from build123d import *

# Parameters (mm, degrees)
BOSS_EXTRUDE1_DEPTH = 10
CUT_EXTRUDE1_DEPTH  = 56.837607918
SKETCH3_R           = 2
CUT_EXTRUDE2_DEPTH  = 3
CUT_EXTRUDE3_DEPTH  = 1.5
FILLET1_R           = 3


with BuildPart() as part:
    # Sketch1 → Boss-Extrude1 (new body)
    with BuildSketch(Plane(origin=(0, 0, 0), x_dir=(0, 0, -1), z_dir=(1, 0, 0))):
        Polygon((0, 0), (0, 45), (31.509339219, 0), align=None)
    extrude(amount=-BOSS_EXTRUDE1_DEPTH)

    # Sketch2 → Cut-Extrude1 (cut, through all)
    with BuildSketch(Plane(origin=(0, 0, 0), x_dir=(0, 0, -1), z_dir=(1, 0, 0))):
        Polygon((25.746392839, 3), (3, 35.485215593), (3, 3), align=None)
    extrude(amount=-CUT_EXTRUDE1_DEPTH, mode=Mode.SUBTRACT)

    # Sketch3 → Cut-Extrude2 (cut)
    with BuildSketch(Plane.XZ):
        with Locations(Location((-5, -8, 0), (0, 0, 270))):
            Circle(SKETCH3_R)
        with Locations(Location((-5, -16, 0), (0, 0, 270))):
            Circle(SKETCH3_R)
    extrude(amount=-CUT_EXTRUDE2_DEPTH, mode=Mode.SUBTRACT)

    # Sketch4 → Cut-Extrude3 (cut)
    with BuildSketch(Plane(origin=(0, 3, 0), x_dir=(1, 0, 0), z_dir=(0, 1, 0))):
        Polygon((-5, 12.025), (-1.55754902, 14.0125), (-1.55754902, 17.9875), (-5, 19.975), (-8.44245098, 17.9875), (-8.44245098, 14.0125), align=None)
        Polygon((-5, 11.975), (-8.44245098, 9.9875), (-8.44245098, 6.0125), (-5, 4.025), (-1.55754902, 6.0125), (-1.55754902, 9.9875), align=None)
    extrude(amount=-CUT_EXTRUDE3_DEPTH, mode=Mode.SUBTRACT)

    # Fillet1
    fillet1_edges = [part.edges().sort_by_distance(p)[0] for p in [
        (-5, 0, -31.509339219),
    ]]
    fillet(fillet1_edges, radius=FILLET1_R)


solid = part.part
Source: CAD feature listing. Evaluate the final solid. Frame: model axes, mm. A direction names the side the tool comes from. Give positions to 0.01 mm unless a question says otherwise; leave off trailing zeros. Write each loop counter-clockwise with the first axis right and the second up, starting at its lowest first coordinate (ties: lowest second). Pieces come first, ordered by that corner, then holes. Notation, with made-up numbers: M -8,66 L 35,66 A14 cw 35,85 Z; hole C -30.5,60.25 d9. An arc over 180 degrees is marked long. Return JSON: item names as keys, results as strings. Group by question number.
1) Pull-direction query (X, two-part tool) for faces 4 (the face through (-6.774, 0.74, -16.923)), 5 (the face through (-5, 19, -3)), 6 (the face through (0, 20.9, -13.4)); classes: pulls with the +X half, pulls with the -X half, needs draft (parallel to the pull), parting line crosses it, or undercut.
2) Set-up query: faces 1 (the face through (-6.745, 2.26, -13.033)), 2 (the face through (-4.93, 25.142, -13.904)), 3 (the face through (-6.2, 0.7, -6.4)). Return all of +Z, -Z, +X, -X, +Y, -Y with unobstructed straight access to the full face (end or side cutting, diameter ignored); none if empty.
3) Cut plane B-B, the plane z = -6.5. Output: boundary loops of the cut face in (x, y).
4) Cut plane A-A, the plane x = -5.5. Output: boundary loops of the cut face in (y, z).
5) Cut plane C-C, the plane y = 17. Output: boundary loops of the cut face in (x, z), plus the area to 3 significant figures.
6) Cut plane D-D, the plane z = -18.5. Output: boundary loops of the cut face in (x, y), plus the area to 3 significant figures.
7) Material intervals for line 1 along X through (y, z) = (0.6, -8); line 2 along Z through (x, y) = (-5, 7); line 3 along Z through (x, y) = (-2.25, 35), sorted ascending. Write a range as [from, to].
8) Pin query (flat end, axial travel): P1, Ø6, axis at x = -8, z = -22.5, coming from the +Y side; P2, Ø4.5, axis at x = -5, z = -8, coming from the +Y side; P3, Ø5.5, axis at x = -6.5, z = -6.5, coming from the +Y side. Return the tip coordinate at first contact, or that it passes through.
Recorded:
{
 "1": {"face 4": "undercut", "face 5": "needs draft", "face 6": "pulls with the +X half"},
 "2": {"face 1": "none", "face 2": "-Z, +X, -X, +Y", "face 3": "-Y"},
 "3": {"outline": "M -10,0 L -6.32,0 L -6.32,1.5 L -8.44,1.5 L -8.44,3 L -10,3 Z; M -10,30.49 L 0,30.49 L 0,35.72 L -10,35.72 Z; M -3.68,0 L 0,0 L 0,3 L -1.56,3 L -1.56,1.5 L -3.68,1.5 Z"},
 "4": {"outline": "M 0,-25.75 A3 ccw 4.72,-28.2 L 45,0 L 0,0 L 0,-6.06 L 1.5,-6.06 L 1.5,-4.31 L 3,-4.31 L 3,-3 L 35.49,-3 L 3,-25.75 L 3,-19.69 L 1.5,-19.69 L 1.5,-17.94 L 0,-17.94 Z; M 0,-14.06 L 1.5,-14.06 L 1.5,-12.31 L 3,-12.31 L 3,-11.69 L 1.5,-11.69 L 1.5,-9.94 L 0,-9.94 Z"},
 "5": {"outline": "M -10,-19.61 L 0,-19.61 L 0,-15.94 L -10,-15.94 Z; M -10,-3 L 0,-3 L 0,0 L -10,0 Z", "area": "66.6 mm²"},
 "6": {"outline": "M -10,0 L 0,0 L 0,3 L -2.45,3 L -2.45,1.5 L -7.55,1.5 L -7.55,3 L -10,3 Z; M -10,13.35 L 0,13.35 L 0,18.58 L -10,18.58 Z", "area": "74.6 mm²"},
 "7": {"line 1": "x = [-10, -7], [-3, 0]", "line 2": "z = [-26.61, -22.95], [-3, 0]", "line 3": "z = [-7, -3.34], [-3, 0]"},
 "8": {"P1": "stops at y = 17.15", "P2": "stops at y = 36.79", "P3": "stops at y = 39.64"}
}
